Check sheet for the modelled part. Datum: model origin and axes. Units: mm. Face numbers are marked on the shaded views. A direction names the side the tool comes from. Give positions to 0.01 mm unless a question says otherwise; leave off trailing zeros. Order: outer loops, then holes, each group sorted by start corner. A loop starts at its lowest first (then second) coordinate and runs counter-clockwise, first axis right, second up.
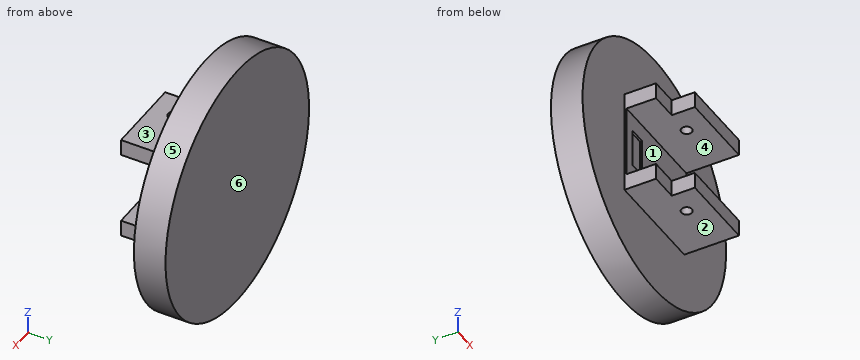
from build123d import *

# Parameters (mm, degrees)
SKETCH1_R           = 12
BOSS_EXTRUDE1_DEPTH = 3
SKETCH3_W           = 10
SKETCH3_H           = 10
BOSS_EXTRUDE3_DEPTH = 3
SKETCH4_R           = 0.5
CUT_EXTRUDE1_DEPTH  = 9
SKETCH5_W           = 3.622801716
SKETCH5_H           = 3
CUT_EXTRUDE2_DEPTH  = 9
BOSS_EXTRUDE5_REACH = 23.024
SKETCH6_W           = 7.376723675
SKETCH6_H           = 5.195198294
SKETCH7_R           = 0.5
CUT_EXTRUDE3_DEPTH  = 14
SKETCH8_W           = 3.773751788
SKETCH8_H           = 4.487553498
CUT_EXTRUDE4_DEPTH  = 22.447379451
SKETCH9_W           = 10
SKETCH9_H           = 6.886875894
CUT_EXTRUDE5_DEPTH  = 5


with BuildPart() as part:
    # Sketch1 → Boss-Extrude1 (new body)
    with BuildSketch(Plane(origin=(0, 0, 0), x_dir=(1, 0, 0), z_dir=(0, 1, 0))):
        with Locations(Location((0, 0, 0), (0, 0, 270))):
            Circle(SKETCH1_R)
    extrude(amount=BOSS_EXTRUDE1_DEPTH)

    # Sketch3 → Boss-Extrude3 (add)
    with BuildSketch(Plane.XZ):
        Rectangle(SKETCH3_W, SKETCH3_H)
    extrude(amount=BOSS_EXTRUDE3_DEPTH)

    # Sketch4 → Cut-Extrude1 (cut)
    with BuildSketch(Plane(origin=(0, 0, -5), x_dir=(-1, 0, 0), z_dir=(0, 0, -1))):
        with Locations((0, -1.5)):
            Circle(SKETCH4_R)
    extrude(amount=-CUT_EXTRUDE1_DEPTH, mode=Mode.SUBTRACT)

    # Sketch5 → Cut-Extrude2 (cut)
    with BuildSketch(Plane(origin=(5, 0, 0), x_dir=(0, 0, -1), z_dir=(1, 0, 0))):
        with Locations((0, -1.5)):
            Rectangle(SKETCH5_W, SKETCH5_H)
    extrude(amount=-CUT_EXTRUDE2_DEPTH, mode=Mode.SUBTRACT)

    # Boss-Extrude5: up to this face of the body (flat: up to its plane)
    boss_extrude5_end = Plane(part.part.faces().sort_by_distance((0, -1.5, 5))[0])
    # Sketch6 → Boss-Extrude5 (add, up to the picked face)
    with BuildSketch(Plane(origin=(0, 0, -5), x_dir=(-1, 0, 0), z_dir=(0, 0, -1)), mode=Mode.PRIVATE) as boss_extrude5_sk1:
        with Locations((-1.311638162, -2.597599147)):
            Rectangle(SKETCH6_W, SKETCH6_H)
    boss_extrude5_tool1 = split(extrude(boss_extrude5_sk1.sketch, amount=-BOSS_EXTRUDE5_REACH, mode=Mode.PRIVATE), bisect_by=boss_extrude5_end, keep=Keep.BOTH, mode=Mode.PRIVATE)
    add(boss_extrude5_tool1.solids().sort_by(Axis((1.311638, -2.597599, -5), (0, 0, 1)))[0])

    # Sketch7 → Cut-Extrude3 (cut)
    with BuildSketch(Plane.XY.offset(5)):
        with Locations((0, -3.072529249)):
            Circle(SKETCH7_R)
    extrude(amount=-CUT_EXTRUDE3_DEPTH, mode=Mode.SUBTRACT)

    # Sketch8 → Cut-Extrude4 (cut, through all)
    with BuildSketch(Plane.ZY.offset(5)):
        with Locations((0, -2.951421545)):
            Rectangle(SKETCH8_W, SKETCH8_H)
    extrude(amount=-CUT_EXTRUDE4_DEPTH, mode=Mode.SUBTRACT)

    # Sketch9 → Cut-Extrude5 (cut)
    with BuildSketch(Plane.XZ.offset(5.195198294)):
        Rectangle(SKETCH9_W, SKETCH9_H)
    extrude(amount=-CUT_EXTRUDE5_DEPTH, mode=Mode.SUBTRACT)


solid = part.part
1) Section check C-C, the plane z = 0. Record the cut outline in (x, y), then the cut area to 3 significant figures.
Recorded:
outline: (-12, 0) - (-5, 0) - (-5, -0.2) - (-4, -0.2) - (-4, 0) - (-2.38, 0) - (-2.38, -0.2) - (5, -0.2) - (5, 0) - (12, 0) - (12, 3) - (-12, 3) - close
area: 73.6 mm2
2) Depth check by flat-ended pin: pin 1 Ø1.7 at (x, z) = (-3, -4) entering from -Y; pin 2 Ø4 at (x, y) = (-4.5, 1) entering from -Z; pin 3 Ø2 at (y, z) = (1.5, -9) entering from +X; pin 4 Ø1.6 at (x, y) = (1, -3.5) entering from -Z. Enter the tip coordinate at first touch or a pass-through.
Recorded:
pin 1: stops at y = -5.2
pin 2: stops at z = -11.74
pin 3: stops at x = 8.94
pin 4: stops at z = -5
3) Set-up check for the marked faces 1, 2 and 3: record each of +Z, -Z, +X, -X, +Y, -Y from which the full face is reachable in a straight line by a thin tool's end or side.
Recorded:
face 1: +X, -X, -Y
face 2: -Z, +X, -X, -Y
face 3: +Z, +X, -X, -Y
4) Section check B-B, the plane x = 0. Record the cut outline in (y, z).
Recorded:
outline: (-5.2, -5) - (-3.57, -5) - (-3.57, -3.44) - (-5.2, -3.44) - close; (-5.2, 3.44) - (-3.57, 3.44) - (-3.57, 5) - (-5.2, 5) - close; (-2.57, -5) - (0, -5) - (0, -12) - (3, -12) - (3, 12) - (0, 12) - (0, 5) - (-2.57, 5) - (-2.57, 3.44) - (-0.2, 3.44) - (-0.2, -3.44) - (-2.57, -3.44) - close
5) Section check D-D, the plane y = -0.5. Record the cut outline in (x, z), then the cut area to 3 significant figures.
Recorded:
outline: (-5, -5) - (5, -5) - (5, -3.44) - (-5, -3.44) - close; (-5, 3.44) - (5, 3.44) - (5, 5) - (-5, 5) - close
area: 31.1 mm2
6) Material ranges on L1, parallel to Y at x = 0, z = 4.4; L2, parallel to Z at x = -2, y = -4.25; L3, parallel to Y at x = -5.5, z = -6.25, recorded low to high.
Recorded:
L1: y = -5.2 to -3.57, -2.57 to 3
L2: z = -5 to -3.44, 3.44 to 5
L3: y = 0 to 3
7) Draft check along Z on the marked faces 4, 5 and 6. Enter one of: +Z half, -Z half, draft (parallel to the pull), parting line (faces both ways), or undercut.
Recorded:
face 4: undercut
face 5: parting line
face 6: draft
8) Section check A-A, the plane y = -4.5. Record the cut outline in (x, z), then the cut area to 3 significant figures.
Recorded:
outline: (-2.38, -5) - (5, -5) - (5, -3.44) - (-2.38, -3.44) - close; (-2.38, 3.44) - (5, 3.44) - (5, 5) - (-2.38, 5) - close
area: 23.0 mm2
